```python
from build123d import *

# Parameters (mm, degrees)
SKETCH1_R           = 5.1
BOSS_EXTRUDE1_DEPTH = 30
FILLET1_R           = 4
CHAMFER1_SIZE       = 2


with BuildPart() as part:
    # Sketch1 → Boss-Extrude1 (new body)
    with BuildSketch(Plane(origin=(0, 0, 0), x_dir=(1, 0, 0), z_dir=(0, 1, 0))):
        with BuildLine():
            Line((3.211102551, 12), (-7, 12))
            Line((-7, 12), (-7, -12))
            Line((-7, -12), (3.211102551, -12))
            ThreePointArc((3.211102551, -12), (10, 0), (3.211102551, 12))
        make_face()
        with Locations(Location((0, 0, 0), (0, 0, 270))):
            Circle(SKETCH1_R, mode=Mode.SUBTRACT)
    extrude(amount=BOSS_EXTRUDE1_DEPTH)

    # Fillet1
    fillet1_edges = [part.edges().sort_by_distance(p)[0] for p in [
        (-7, 15, 12),
        (-7, 15, -12),
    ]]
    fillet(fillet1_edges, radius=FILLET1_R)

    # Chamfer1
    # the kernel refuses this chamfer: 57.143323993, 2 mm, written as the material it takes off along each edge
    with BuildSketch(Plane(origin=(3.211102551, -18.277403027, -12), x_dir=(-1, 0, 0), z_dir=(0, 1, 0))) as chamfer1_piece_1:
        with BuildLine():
            Line((CHAMFER1_SIZE, 0), (-3.792467803, 3.344282846))
            ThreePointArc((-3.792467803, 3.344282846), (-2.856773862, 2.271800551), (0, 0))
            Line((0, 0), (CHAMFER1_SIZE, 0))
        make_face()
    extrude(amount=66.554806053, mode=Mode.SUBTRACT)


solid = part.part
```
Design review of the part built by this model. Coordinates are the model's own, in mm. Give positions to 0.01 mm unless a question says otherwise; leave off trailing zeros. Write each loop counter-clockwise with the first axis right and the second up, starting at its lowest first coordinate (ties: lowest second). Pieces come first, ordered by that corner, then holes. Notation, with made-up numbers: (28, 82.5) -> (73, 82.5) arc R17 cw to (73, 108.5) -> close; hole circle Ø4 at (-14.5, 40). An arc over 180 degrees is marked (long way). Answer in a Markdown table with one row per item.
(1) Consider section D-D (x = 7.5). State the section outline as (y, z) points.
Results:
| item | result |
|---|---|
| outline | (0, -7.98) -> (30, -7.98) -> (30, 7.98) -> (0, 7.98) -> close |
(2) Consider section B-B (z = 0). State the section outline as (x, y) points, then the cut area to 3 significant figures.
Results:
| item | result |
|---|---|
| outline | (-7, 0) -> (-5.1, 0) -> (-5.1, 30) -> (-7, 30) -> close; (5.1, 0) -> (10, 0) -> (10, 30) -> (5.1, 30) -> close |
| area | 204 mm2 |
(3) To check wall thickness, follow probe 1 along X at (y, z) = (18, 0); probe 2 along X at (y, z) = (3.75, 2.75); probe 3 along Z at (x, y) = (-1.5, 2.5). State the ranges of each line that lie inside material, in increasing order.
Results:
| item | result |
|---|---|
| probe 1 | -7 to -5.1, 5.1 to 10 |
| probe 2 | -7 to -4.3, 4.3 to 9.73 |
| probe 3 | -12 to -4.87, 4.87 to 12 |
(4) Consider section C-C (x = 0). State the section outline as (y, z) points.
Results:
| item | result |
|---|---|
| outline | (0, -12) -> (30, -12) -> (30, -5.1) -> (0, -5.1) -> close; (0, 5.1) -> (30, 5.1) -> (30, 12) -> (0, 12) -> close |
(5) Consider section A-A (y = 14). State the section outline as (x, z) points, then the cut area to 3 significant figures.
Results:
| item | result |
|---|---|
| outline | (-7, -8) arc R4 ccw to (-3, -12) -> (1.21, -12) -> (7, -8.66) arc R14 ccw to (3.21, 12) -> (-3, 12) arc R4 ccw to (-7, 8) -> close; hole circle Ø10.2 at (0, 0) |
| area | 268 mm2 |
(6) Mouldability with a two-part tool opening along X and no side actions: class faces 1 (the flat face through (-7, 15, 0)), 2 (the flat face through (4.07, 14.79, -10.35)), 3 (the cylindrical face through (1.532, 14.79, 4.864)) as +X half, -X half, draft (parallel to the pull), parting line (faces both ways), or undercut.
Results:
| item | result |
|---|---|
| face 1 | -X half |
| face 2 | +X half |
| face 3 | undercut |
(7) Clearance check with flat-ended pins moving along their axes: pin 1 (1 mm diameter, centred on x = 5, y = 25.5, fed in from +Z); pin 2 (3 mm diameter, centred on y = 24.5, z = -2, fed in from +X); pin 3 (6 mm diameter, centred on x = -1, z = -6.5, fed in from -Y); pin 4 (6 mm diameter, centred on x = 0, z = 0, fed in from +Y). State where each tip first meets the part, or that it passes through.
Results:
| item | result |
|---|---|
| pin 1 | z = 11.12 |
| pin 2 | x = 9.99 |
| pin 3 | y = 0 |
| pin 4 | through |
